Verification items for the finished model (mm, model axes). Face numbers are marked on the shaded views. A direction names the side the tool comes from. Give positions to 0.01 mm unless a question says otherwise; leave off trailing zeros. Write each loop counter-clockwise with the first axis right and the second up, starting at its lowest first coordinate (ties: lowest second). Pieces come first, ordered by that corner, then holes. Notation, with made-up numbers: (86, -11.5) - (110, -11.5) arc R25 ccw to (110, 22.5) - close; hole circle Ø11 at (33, 73). An arc over 180 degrees is marked (long way). Put each result on its own line as item: value.
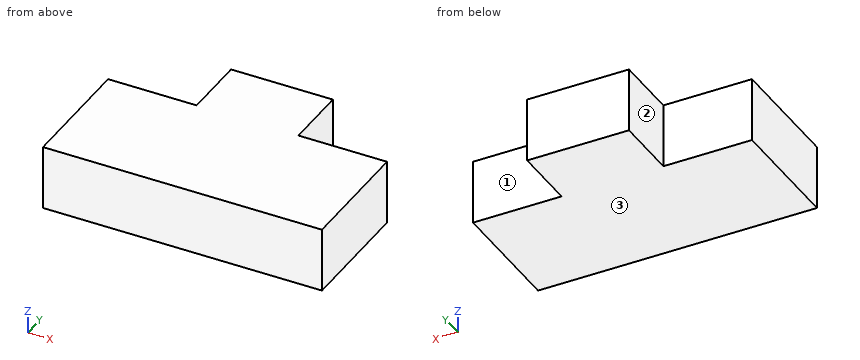
from build123d import *

# Parameters (mm, degrees)
SKETCH1_W           = 27.4
SKETCH1_H           = 6.35
BOSS_EXTRUDE1_DEPTH = 12
SKETCH2_W           = 10
SKETCH2_H           = 6.35
BOSS_EXTRUDE2_DEPTH = 6.35


with BuildPart() as part:
    # Sketch1 → Boss-Extrude1 (new body)
    with BuildSketch(Plane(origin=(0, 0, 0), x_dir=(1, 0, 0), z_dir=(0, 1, 0))):
        with Locations((13.7, 3.175)):
            Rectangle(SKETCH1_W, SKETCH1_H)
    extrude(amount=BOSS_EXTRUDE1_DEPTH)

    # Sketch2 → Boss-Extrude2 (add)
    with BuildSketch(Plane.XY):
        with Locations((13.7, 15.175)):
            Rectangle(SKETCH2_W, SKETCH2_H)
    extrude(amount=-BOSS_EXTRUDE2_DEPTH)


solid = part.part
Q1. Go/stop test with flat-tipped pins: pin 1 Ø1.9 at (y, z) = (15.5, -2) entering from -X; pin 2 Ø1.9 at (y, z) = (14.5, -3) entering from +X; pin 3 Ø1.5 at (x, z) = (10, -3) entering from -Y; pin 4 Ø4 at (x, y) = (22, 14.5) entering from -Z. Record where each tip stops, or that it passes through.
Answers follow:
pin 1: stops at x = 8.7
pin 2: stops at x = 18.7
pin 3: stops at y = 0
pin 4: passes through
Q2. Set-up check for the marked faces 1, 2 and 3: record each of +Z, -Z, +X, -X, +Y, -Y from which the full face is reachable in a straight line by a thin tool's end or side.
Answers follow:
face 1: +Z, -Z, +X, +Y
face 2: +Z, -Z, -X, +Y
face 3: -Z, +X, -X, +Y, -Y
Q3. Scan lines: line 1 along Y through (x, z) = (22.5, -0.25); line 2 along X through (y, z) = (13.5, -0.75). Record each from-to range of solid material in increasing order.
Answers follow:
line 1: y = 0 to 12
line 2: x = 8.7 to 18.7
Q4. Section check A-A, the plane z = -0.5. Record the cut outline in (x, y), plus the area to 3 significant figures.
Answers follow:
outline: (0, 0) - (27.4, 0) - (27.4, 12) - (18.7, 12) - (18.7, 18.35) - (8.7, 18.35) - (8.7, 12) - (0, 12) - close
area: 392 mm2
Q5. Section check B-B, the plane y = 12.75. Record the cut outline in (x, z), plus the area to 3 significant figures.
Answers follow:
outline: (8.7, -6.35) - (18.7, -6.35) - (18.7, 0) - (8.7, 0) - close
area: 63.5 mm2
Q6. Section check C-C, the plane x = 21. Record the cut outline in (y, z).
Answers follow:
outline: (0, -6.35) - (12, -6.35) - (12, 0) - (0, 0) - close
